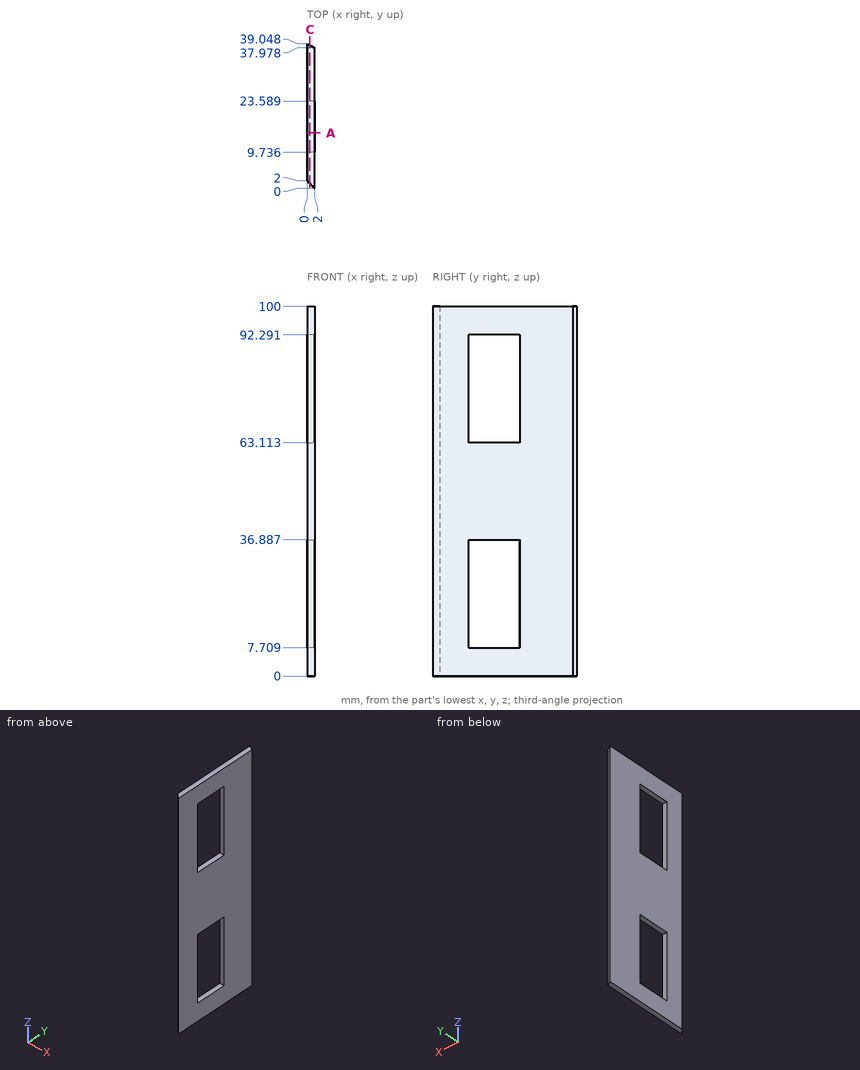
The figure shows three views and two pictorial views of one solid part (mm, origin at its lowest corner). Answer the questions. Give positions to 0.01 mm unless a question says otherwise; leave off trailing zeros. Loops run counter-clockwise (first coordinate to the right, second up) from the corner with the lowest first, then second, coordinate; pieces in that order, holes last. Notation, with made-up numbers: (27, 68) -> (34, 68) arc R12 ccw to (34, 85) -> close; hole circle Ø6 at (-27.75, -36.75). An arc over 180 degrees is marked (long way). Use a Markdown table: item, result. Add a question column.
1. Find the intervals of material crossed by probe 1 along Z at (x, y) = (1.7, 10.5); probe 2 along Y at (x, z) = (1.5, 22) (1 decimal); probe 3 along Y at (x, z) = (0.1, 28) (1 decimal), in increasing order.
2. Flat-ended cylindrical pins translate along their axes: pin 1 Ø1 at (x, y) = (0.5, 15.5) entering from -Z; pin 2 Ø0.6 at (x, z) = (1.5, 22) entering from -Y; pin 3 Ø1 at (x, z) = (0.5, 40.5) entering from -Y; pin 4 Ø0.6 at (x, z) = (0.5, 22) entering from +Y. Find the tip coordinate at first contact, or state that the pin passes through.
3. Section A-A on y = 15 is taken. Determine the outline of the cut face in (x, z).
4. Section C-C on x = 0.75 is taken. State how many separate pieces and enclosed holes the cut face has, and give its area (3 significant figures).
Results below:
| question | item | result |
|---|---|---|
| 1 | probe 1 | z = 0 to 7.71, 36.89 to 63.11, 92.29 to 100 |
| 1 | probe 2 | y = 0.5 to 9.7, 23.6 to 38.2 |
| 1 | probe 3 | y = 1.9 to 9.7, 23.6 to 39 |
| 2 | pin 1 | stops at z = 0 |
| 2 | pin 2 | stops at y = 0.2 |
| 2 | pin 3 | stops at y = 1 |
| 2 | pin 4 | stops at y = 38.94 |
| 3 | outline | (0, 0) -> (2, 0) -> (2, 7.71) -> (0, 7.71) -> close; (0, 36.89) -> (2, 36.89) -> (2, 63.11) -> (0, 63.11) -> close; (0, 92.29) -> (2, 92.29) -> (2, 100) -> (0, 100) -> close |
| 4 | separate pieces | 1 |
| 4 | enclosed holes | 2 |
| 4 | area | 2,930 mm^2 |
